Input: part model. Units: mm. Frame: model coordinates. A direction names the side the tool comes from. Coordinates: 2 decimals unless noted, no trailing zeros. Order: outer loops, then holes, each group sorted by start corner. A loop starts at its lowest first (then second) coordinate and runs counter-clockwise, first axis right, second up.
Autodesk Inventor part; units mm, degrees
ref_plane "YZ Plane" through (0, 0, 0) normal (1, 0, 0) x (0, 1, 0)
ref_plane "XZ Plane" through (0, 0, 0) normal (0, 1, 0) x (-1, 0, 0)
ref_plane "XY Plane" through (0, 0, 0) normal (0, 0, 1) x (1, 0, 0)
sketch "Sketch1" plane through (0, 0, 0) normal (0, 0, 1) x (1, 0, 0)
  circle A0 centre (0, 0) radius 13.8
  circle A1 centre (0, 0) radius 11.5
  circle A2 centre (0, 0) radius 15.6
  circle A3 centre (0, 0) radius 12.5
  dimension "d0" = 27.6
  dimension "d1" = 23
  dimension "d2" = 31.2
  dimension "d3" = 25
extrude "Extrusion1" add sketch "Sketch1" along normal blind 1 contours A3
extrude "Extrusion2" add sketch "Sketch1" along normal blind 3 contours A0
sketch "Sketch2" plane through (0, 0, 3) normal (0, 0, 1) x (1, 0, 0)
  circle A0 centre (0, 0) radius 15.6
  circle A1 centre (0, 0) radius 12.5
extrude "Extrusion3" add sketch "Sketch2" along normal blind 1
sketch "Sketch4" plane through (0, 0, 4) normal (0, 0, 1) x (1, 0, 0)
  circle A0 centre (0, 0) radius 16
  circle A1 centre (0, 0) radius 17
  circle A2 centre (0, 0) radius 12.5
  dimension "d14" = 32
  dimension "d15" = 34
extrude "Extrusion5" add sketch "Sketch4" along normal blind 0.5 contours A0
extrude "Extrusion6" add sketch "Sketch4" along normal blind 4 contours A1
sketch "Sketch8" plane through (0, 0, 8) normal (0, 0, 1) x (1, 0, 0)
  line L0 (0.5, 10) -> (-0.5, 10)
  line L1 (-0.5, 10) -> (-0.5, 20)
  line L2 (-0.5, 20) -> (0.5, 20)
  line L3 (0.5, 20) -> (0.5, 10)
  circle A0 centre (0, 0) radius 15
  line L4 (0.5, 10) -> (-0.5, 20) construction
  line L5 (-0.5, 10) -> (0.5, 20) construction
  point P0 (0, 15)
  dimension "d30" = 1
  dimension "d31" = 10
extrude "Extrusion10" cut sketch "Sketch8" against normal blind 10 contours L0 L1 A0 L3 | A0 L1 L2 L3 picked at (-0.0556, 11.6664)
properties part number "32to25mmFilterAdapter"
Item 1: Ray query, probe 1 along X at (y, z) = (0, 3.55); probe 2 along X at (y, z) = (0, 2.8); probe 3 along Y at (x, z) = (-10.5, 2). Return the intervals inside material, ascending.
Response values:
probe 1: x = -15.6 to -12.5, 12.5 to 15.6
probe 2: x = -13.8 to -12.5, 12.5 to 13.8
probe 3: y = -8.95 to -6.78, 6.78 to 8.95
Item 2: Cut plane D-D on z = 2.25. Return loops of the section in (x, y).
Response values:
outline: (-0.5, 12.49) - (-0.5, 13.79) arc R13.8 ccw (long way) to (0.5, 13.79) - (0.5, 12.49) arc R12.5 cw (long way) to start
Item 3: Access query for faces 1 (the face through (-8, -14, 4)), 2 (the face through (-0.5, 14, 4)), 3 (the face through (-9.3, -7.1, 0)). Directions: +Z, -Z, +X, -X, +Y, -Y. A direction counts if a zero-diameter tool reaches every point of the face in a straight line with its end or side. Return the directions, or none.
Response values:
face 1: -Z
face 2: +Z, -Z, +Y
face 3: -Z, +X, -X, +Y, -Y
Item 4: Cut plane A-A on x = 0. Return loops of the section in (y, z), then the cut area to 4 significant figures.
Response values:
outline: (-17, 4) - (-15.6, 4) - (-15.6, 3) - (-13.8, 3) - (-13.8, 0) - (-11.5, 0) - (-11.5, 1) - (-12.5, 1) - (-12.5, 4.5) - (-16, 4.5) - (-16, 8) - (-17, 8) - close
area: 13.75 mm2
Item 5: Pin query (flat end, axial travel): pin 1 Ø1 at (y, z) = (-12.5, 6) entering from +X; pin 2 Ø4.5 at (y, z) = (14.5, 4) entering from -X; pin 3 Ø4.5 at (y, z) = (14, 5) entering from +X. Return the tip coordinate at first contact, or that it passes through.
Response values:
pin 1: stops at x = 12.04
pin 2: stops at x = -11.79
pin 3: stops at x = 12.29
Item 6: Draft query along Y for faces 4 (the face through (-6, -10, 1)), 5 (the face through (1, -14, 3)), 6 (the face through (-10, 8, 4.5)). Return one class per face: pulls with the +Y half, pulls with the -Y half, needs draft (parallel to the pull), parting line crosses it, or undercut.
Response values:
face 4: undercut
face 5: needs draft
face 6: undercut
Item 7: Cut plane B-B on y = 8. Return loops of the section in (x, z), then the cut area to 3 significant figures.
Response values:
outline: (-15, 4) - (-13.39, 4) - (-13.39, 3) - (-11.24, 3) - (-11.24, 0) - (-8.26, 0) - (-8.26, 1) - (-9.6, 1) - (-9.6, 4.5) - (-13.86, 4.5) - (-13.86, 8) - (-15, 8) - close; (8.26, 0) - (11.24, 0) - (11.24, 3) - (13.39, 3) - (13.39, 4) - (15, 4) - (15, 8) - (13.86, 8) - (13.86, 4.5) - (9.6, 4.5) - (9.6, 1) - (8.26, 1) - close
area: 33.5 mm2
Item 8: Cut plane C-C on x = -5.5. Return loops of the section in (y, z), then the cut area to 3 significant figures.
Response values:
outline: (-16.09, 4) - (-14.6, 4) - (-14.6, 3) - (-12.66, 3) - (-12.66, 0) - (-10.1, 0) - (-10.1, 1) - (-11.22, 1) - (-11.22, 4.5) - (-15.02, 4.5) - (-15.02, 8) - (-16.09, 8) - close; (10.1, 0) - (12.66, 0) - (12.66, 3) - (14.6, 3) - (14.6, 4) - (16.09, 4) - (16.09, 8) - (15.02, 8) - (15.02, 4.5) - (11.22, 4.5) - (11.22, 1) - (10.1, 1) - close
area: 29.9 mm2
